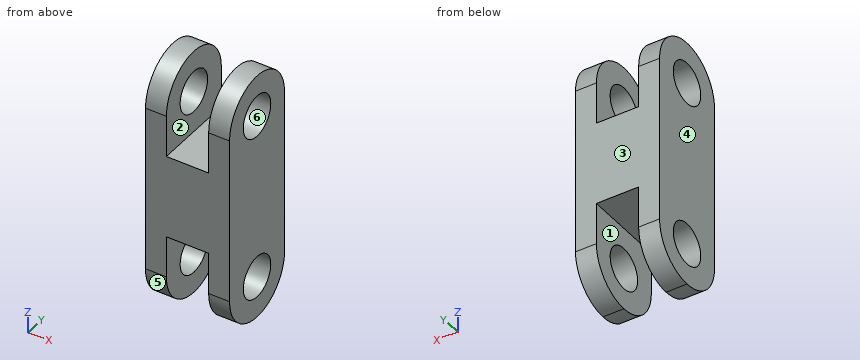
```python
from build123d import *

# Parameters (mm, degrees)
F0_W     = 40
F0_H     = 80
F1_DEPTH = 20.1
F2_R     = 10
F3_DEPTH = 10
F5_W     = 20.2
F5_H     = 40
F6_DEPTH = 40
F7_R     = 10
F8_DEPTH = 40.2
F9_R     = 19.99999


# Not quite as in the source:
# - a fillet or chamfer is up to 0.001 mm smaller than in the source, because OpenCascade refuses the exact size


with BuildPart() as f1:
    # F0 (on Right) → F1 (new body)
    with BuildSketch(Plane.YZ):
        Rectangle(F0_W, F0_H)
    extrude(amount=F1_DEPTH)

    # F2 (on face) → F3 (join)
    with BuildSketch(Plane.YZ.offset(20.1)):
        with BuildLine():
            Line((-20, 60), (-20, 40))
            Line((-20, 40), (20, 40))
            Line((20, 40), (20, 60))
            ThreePointArc((20, 60), (0, 80), (-20, 60))
        make_face()
        with Locations((0, 60)):
            Circle(F2_R, mode=Mode.SUBTRACT)
    extrude(amount=-F3_DEPTH)

    # F4: F1 across face


with BuildPart() as f1_1:
    add(f1.part)
    add(f1.part.mirror(Plane(origin=(0, 0, 0), x_dir=(0, 1, 0), z_dir=(-1, 0, 0))))

    # F5 (on face) → F6 (cut, through all)
    with BuildSketch(Plane.XZ.offset(20)):
        with Locations((0, -20)):
            Rectangle(F5_W, F5_H)
    extrude(amount=-F6_DEPTH, mode=Mode.SUBTRACT)

    # F7 (on face) → F8 (cut, through all)
    with BuildSketch(Plane.YZ.offset(20.1)):
        with Locations((0, -20)):
            Circle(F7_R)
    extrude(amount=-F8_DEPTH, mode=Mode.SUBTRACT)

    # F9 (radius 20 in the source; OpenCascade refuses exactly that, so slightly less here)
    f9_edges = [f1_1.edges().sort_by_distance(p)[0] for p in [
        (-15.1, 20, -40),
        (-15.1, -20, -40),
        (15.1, 20, -40),
        (15.1, -20, -40),
    ]]
    fillet(f9_edges, radius=F9_R)


solid = f1_1.part
```
CAD build for the part. Positions are in the model's coordinates, mm. Face numbers are marked on the shaded views. A direction names the side the tool comes from. Round coordinates to 2 decimals unless told otherwise and drop trailing zeros. Loops run counter-clockwise (first coordinate to the right, second up) from the corner with the lowest first, then second, coordinate; pieces in that order, holes last. Notation, with made-up numbers: M 8,80.5 L 45,80.5 A23 cw 45,108.5 Z; hole C 17,70 d10. An arc over 180 degrees is marked long. Return JSON: item names as keys, results as strings. Group by question number.
(1) Saw through at B-B, the plane x = -18. Give the number of separate pieces and of enclosed holes in the cut face, and give its area (3 significant figures).
(2) Tool access for the marked faces 1, 2 and 3: list every direction of +Z, -Z, +X, -X, +Y, -Y with a clear straight run to the whole face (end or side of a thin tool).
(3) Saw through at D-D, the plane y = 16. List the corners of the cut face in (x, z).
(4) Drop flat-ended pins along their axis: P1, Ø6, axis at x = -1.5, y = -3, coming from the +Z side; P2, Ø3, axis at x = 5, y = 13, coming from the -Z side; P3, Ø8, axis at x = -15, y = -14.5, coming from the -Z side. Give the stop position or say it passes through.
(5) Saw through at C-C, the plane y = -3. List the corners of the cut face in (x, z).
(6) Wall check: probe 1 along Z at (x, y) = (-13, 0); probe 2 along X at (y, z) = (-17, -8); probe 3 along Z at (x, y) = (-17, -6). Give the ranges that are in metal, low to high. Write a range as [from, to].
(7) Mould opens along Z. For the marked faces 4, 5 and 6 say: +Z half, -Z half, draft (parallel to the pull), parting line (faces both ways), or undercut.
(8) Saw through at A-A, the plane z = -12. List the corners of the cut face in (x, y).
Answer list:
{
 "1": {"separate pieces": "1", "enclosed holes": "2", "area": "3,830 mm2"},
 "2": {"face 1": "-Z, +Y, -Y", "face 2": "+Z, +Y, -Y", "face 3": "+Z, -Z, +X, -X, +Y"},
 "3": {"outline": "M -20.1,-32 L -10.1,-32 L -10.1,0 L 10.1,0 L 10.1,-32 L 20.1,-32 L 20.1,72 L 10.1,72 L 10.1,40 L -10.1,40 L -10.1,72 L -20.1,72 Z"},
 "4": {"P1": "z = 40", "P2": "z = 0", "P3": "z = -37.02"},
 "5": {"outline": "M -20.1,-39.77 L -10.1,-39.77 L -10.1,-29.54 L -20.1,-29.54 Z; M -20.1,-10.46 L -10.1,-10.46 L -10.1,0 L 10.1,0 L 10.1,-10.46 L 20.1,-10.46 L 20.1,50.46 L 10.1,50.46 L 10.1,40 L -10.1,40 L -10.1,50.46 L -20.1,50.46 Z; M -20.1,69.54 L -10.1,69.54 L -10.1,79.77 L -20.1,79.77 Z; M 10.1,-39.77 L 20.1,-39.77 L 20.1,-29.54 L 10.1,-29.54 Z; M 10.1,69.54 L 20.1,69.54 L 20.1,79.77 L 10.1,79.77 Z"},
 "6": {"probe 1": "[-40, -30], [-10, 50], [70, 80]", "probe 2": "[-20.1, -10.1], [10.1, 20.1]", "probe 3": "[-39.08, -28], [-12, 52], [68, 79.08]"},
 "7": {"face 4": "draft", "face 5": "-Z half", "face 6": "undercut"},
 "8": {"outline": "M -20.1,-20 L -10.1,-20 L -10.1,-6 L -20.1,-6 Z; M -20.1,6 L -10.1,6 L -10.1,20 L -20.1,20 Z; M 10.1,-20 L 20.1,-20 L 20.1,-6 L 10.1,-6 Z; M 10.1,6 L 20.1,6 L 20.1,20 L 10.1,20 Z"}
}
